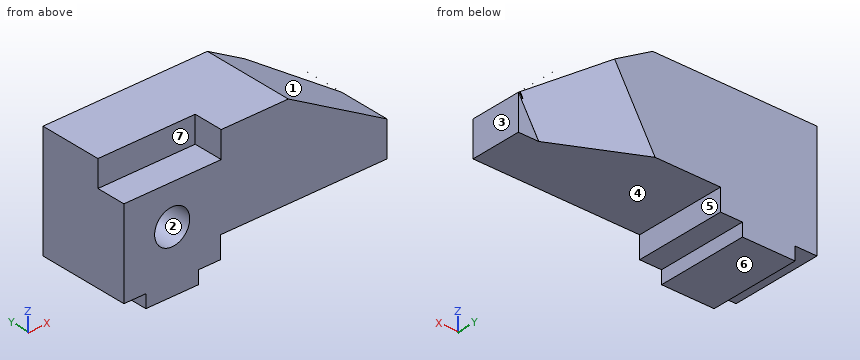
```python
from build123d import *

# Parameters (mm, degrees)
F0_W      = 44
F0_H      = 30
F1_DEPTH  = 42
F3_D      = 16
F3_DEPTH  = 22
F3_TIP    = 4.8068849522
F4_W      = 44.3841926754
F4_H      = 12
F5_DEPTH  = 13.5
F8_DEPTH  = 87.7304734195
F10_DEPTH = 18.45
F11_DEPTH = 0.6


with BuildPart() as f1:
    # F0 (on Front) → F1 (new body)
    with BuildSketch(Plane.XZ):
        with Locations((22, 15)):
            Rectangle(F0_W, F0_H)
        Polygon((44, 0), (0, 0), (0, -10), (10, -10), (10, -16), (34, -16), (34, -10), (44, -10), align=None)
        Polygon((44, 30), (44, 0), (120, 0), (120, 16.0192378865), (75, 42), (0, 42), (0, 30), align=None)
    extrude(amount=F1_DEPTH)

    # F3
    with Locations(Plane.XZ.offset(42)):
        with Locations((22, 12)):
            Hole(F3_D / 2, depth=F3_DEPTH)
            with Locations((0, 0, -(F3_DEPTH + F3_TIP / 2))):  # 118° drill point
                Cone(0, F3_D / 2, F3_TIP, mode=Mode.SUBTRACT)

    # F4 (on face) → F5 (cut)
    with BuildSketch(Plane.XZ.offset(42)):
        with Locations((22.1920963377, 36)):
            Rectangle(F4_W, F4_H)
    extrude(amount=-F5_DEPTH, mode=Mode.SUBTRACT)

    # F7 (on face) → F8 (cut, through all)
    with BuildSketch(Plane(origin=(36.9365334795, 0, 63.9759526419), x_dir=(0.8660254038, 0, -0.5), z_dir=(0.5, 0, 0.8660254038))):
        Polygon((95.9134295109, 0), (63.9519052838, 0), (95.9134295109, -18.4529946162), align=None)
    extrude(amount=-F8_DEPTH, mode=Mode.SUBTRACT)

    # F9 (on face) → F10 (cut)
    with BuildSketch(Plane.XZ):
        Polygon((120.1416030526, 0), (120.0014874339, 16.0108022392), (110.7117310166, 0), align=None)
    extrude(amount=F10_DEPTH, mode=Mode.SUBTRACT)

    # F11 (cut): faces of the model
    f11_faces = [f1.faces().sort_by_distance(p)[0] for p in [
        (112.9756224533, -18.4444052592, 3.9017942404),
        (119.3575829171, -9.225, 14.9010392468),
    ]]
    extrude(f11_faces, amount=-F11_DEPTH, mode=Mode.SUBTRACT)


solid = f1.part
```
Work out the finished part from the listing and answer in its coordinate system (mm). Face numbers are marked on the shaded views. A direction names the side the tool comes from. Give positions to 0.01 mm unless a question says otherwise; leave off trailing zeros. Loops run counter-clockwise (first coordinate to the right, second up) from the corner with the lowest first, then second, coordinate; pieces in that order, holes last. Notation, with made-up numbers: (10.25, 30) -> (28.25, 30) arc R30 ccw to (28.25, 61) -> close; hole circle Ø5 at (64.25, 50.25). An arc over 180 degrees is marked (long way). One line per question, with ' | ' between items. Start each with the question number.
1) Each of these flat-tipped pins is pushed along its axis until it touches: pin 1 (8 mm diameter, centred on y = -5.5, z = 31, fed in from +X); pin 2 (2 mm diameter, centred on x = 113.5, z = 9, fed in from +Y); pin 3 (3 mm diameter, centred on x = 4, y = -30.5, fed in from -Z). Where does it stop, or does it pass through?
2) For the marked faces 5, 6 and 7, determine the directions among +Z, -Z, +X, -X, +Y, -Y from which every point of the face is accessible in a straight line to the end or side of a thin tool.
3) Section A-A, the plane y = -35 is taken. Determine the outline of the cut face in (x, z), then the cut area to 3 significant figures.
4) Section B-B, the plane x = 38 is taken. Determine the outline of the cut face in (y, z).
5) Determine the mould class of the marked faces 1, 2, 3 and 4 for opening direction Z: +Z half, -Z half, draft (parallel to the pull), parting line (faces both ways), or undercut.
6) Straight lines are drawn through the part: L1, parallel to X at y = -28.75, z = 12; L2, parallel to Z at x = 22, y = -29; L3, parallel to Y at x = 30, z = 37. For each, find the intervals that lie inside material, in ascending order.
Resolved:
1) pin 1: x = 100.97 | pin 2: y = -16.65 | pin 3: z = -10
2) face 5: -Z, +X, +Y, -Y | face 6: -Z, +X, -X, +Y, -Y | face 7: +Z, -X, -Y
3) outline: (0, -10) -> (10, -10) -> (10, -16) -> (34, -16) -> (34, -10) -> (44, -10) -> (44, 0) -> (120, 0) -> (120, 16.02) -> (75, 42) -> (44.38, 42) -> (44.38, 30) -> (0, 30) -> close; hole circle Ø16 at (22, 12) | area: 4,310 mm2
4) outline: (-42, -10) -> (0, -10) -> (0, 42) -> (-28.5, 42) -> (-28.5, 30) -> (-42, 30) -> close
5) face 1: +Z half | face 2: undercut | face 3: draft | face 4: -Z half
6) L1: 0 to 14, 30 to 120 | L2: -16 to 4, 20 to 30 | L3: -28.5 to 0
